Verification items for the finished model (mm, model axes). Face numbers are marked on the shaded views. A direction names the side the tool comes from. Give positions to 0.01 mm unless a question says otherwise; leave off trailing zeros. Order: outer loops, then holes, each group sorted by start corner. A loop starts at its lowest first (then second) coordinate and runs counter-clockwise, first axis right, second up.
from build123d import *

# Parameters (mm, degrees)
ESQUISSE1_W                                    = 41
ESQUISSE1_H                                    = 72
ESQUISSE1_W_2                                  = 21
ESQUISSE1_H_2                                  = 21
BOSS_EXTRU_1_DEPTH                             = 10
ESQUISSE3_W                                    = 10
ESQUISSE3_H                                    = 10
BOSS_EXTRU_2_DEPTH                             = 20
FRAISAGE_POUR_VIS_T_TE_FRAIS_E_M31_D           = 3.4
FRAISAGE_POUR_VIS_T_TE_FRAIS_E_M31_CSINK_D     = 6.3
FRAISAGE_POUR_VIS_T_TE_FRAIS_E_M31_CSINK_ANGLE = 90
CONG_2_R                                       = 10
CONG_3_R                                       = 5
CONG_4_R                                       = 10


with BuildPart() as part:
    # Esquisse1 → Boss.-Extru.1 (new body)
    with BuildSketch(Plane.XY):
        with Locations((20.5, 36)):
            Rectangle(ESQUISSE1_W, ESQUISSE1_H)
        with Locations((20.5, 51.5)):
            Rectangle(ESQUISSE1_W_2, ESQUISSE1_H_2, mode=Mode.SUBTRACT)
    extrude(amount=BOSS_EXTRU_1_DEPTH)

    # Esquisse3 → Boss.-Extru.2 (add)
    with BuildSketch(Plane.XY.offset(10)):
        with Locations((36, 5)):
            Rectangle(ESQUISSE3_W, ESQUISSE3_H)
        with Locations((5, 5)):
            Rectangle(ESQUISSE3_W, ESQUISSE3_H)
    extrude(amount=BOSS_EXTRU_2_DEPTH)

    # Fraisage pour vis à tête fraisée M31 (through all)
    with Locations(Plane(origin=(0, 10, 0), x_dir=(1, 0, 0), z_dir=(0, 1, 0))):
        with Locations((5, -25.5), (36, -25.5)):
            CounterSinkHole(FRAISAGE_POUR_VIS_T_TE_FRAIS_E_M31_D / 2, FRAISAGE_POUR_VIS_T_TE_FRAIS_E_M31_CSINK_D / 2, counter_sink_angle=FRAISAGE_POUR_VIS_T_TE_FRAIS_E_M31_CSINK_ANGLE)

    # Congé2
    cong_2_edges = [part.edges().sort_by_distance(p)[0] for p in [
        (0, 72, 5),
        (41, 72, 5),
    ]]
    fillet(cong_2_edges, radius=CONG_2_R)

    # Congé3
    cong_3_edges = [part.edges().sort_by_distance(p)[0] for p in [
        (10, 5, 10),
        (31, 5, 10),
        (41, 5, 30),
        (31, 5, 30),
        (10, 5, 30),
        (0, 5, 30),
    ]]
    fillet(cong_3_edges, radius=CONG_3_R - 0.0001)  # a hair under: the kernel refuses the full size

    # Congé4
    cong_4_edges = [part.edges().sort_by_distance(p)[0] for p in [
        (33.50005, 10, 10),
        (7.49995, 10, 10),
    ]]
    fillet(cong_4_edges, radius=CONG_4_R)


solid = part.part
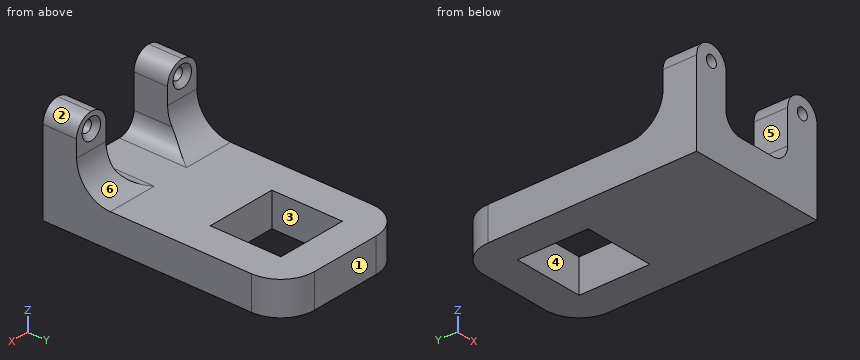
(1) Go/stop test with flat-tipped pins: pin 1 (2 mm diameter, centred on x = 32.5, y = 34.5, fed in from +Z); pin 2 (5 mm diameter, centred on x = 36, z = 23.5, fed in from +Y); pin 3 (1 mm diameter, centred on x = 8, z = 13.5, fed in from +Y). Record where each tip stops, or that it passes through.
Solved:
pin 1: stops at z = 10
pin 2: stops at y = 10
pin 3: stops at y = 12.86
(2) Section check A-A, the plane z = 21. Enter the section's corners in (x, y).
Solved:
outline: (0, 0) - (10, 0) - (10, 10) - (0, 10) - close; (31, 0) - (41, 0) - (41, 10) - (31, 10) - close
(3) Release check for a two-part mould opening along Y. For the marked faces 1, 2 and 3 record: pulls with the +Y half, pulls with the -Y half, needs draft (parallel to the pull), parting line crosses it, or undercut.
Solved:
face 1: pulls with the +Y half
face 2: needs draft
face 3: undercut
(4) Scan lines: line 1 (Z direction, x = 36, y = 4); line 2 (X direction, y = 53.5, z = 8.25); line 3 (X direction, y = 2, z = 25.5). Record each from-to range of solid material in increasing order.
Solved:
line 1: z = 0 to 23.8, 27.2 to 30
line 2: x = 0 to 10, 31 to 41
line 3: x = 0.03 to 3.3, 6.7 to 9.97, 31.03 to 34.3, 37.7 to 40.97
(5) Section check D-D, the plane y = 67. Enter the section's corners in (x, z), then the cut area to 3 significant figures.
Solved:
outline: (1.34, 0) - (39.66, 0) - (39.66, 10) - (1.34, 10) - close
area: 383 mm2
(6) Section check C-C, the plane y = 30. Enter the section's corners in (x, z), then the cut area to 3 significant figures.
Solved:
outline: (0, 0) - (41, 0) - (41, 10) - (0, 10) - close
area: 410 mm2
(7) Section check B-B, the plane x = 25. Enter the section's corners in (y, z).
Solved:
outline: (0, 0) - (41, 0) - (41, 10) - (0, 10) - close; (62, 0) - (72, 0) - (72, 10) - (62, 10) - close
(8) Set-up check for the marked faces 4, 5 and 6: record each of +Z, -Z, +X, -X, +Y, -Y from which the full face is reachable in a straight line by a thin tool's end or side.
Solved:
face 4: +Z, -Z
face 5: +Z, +Y, -Y
face 6: +Z, +X, -X, +Y
